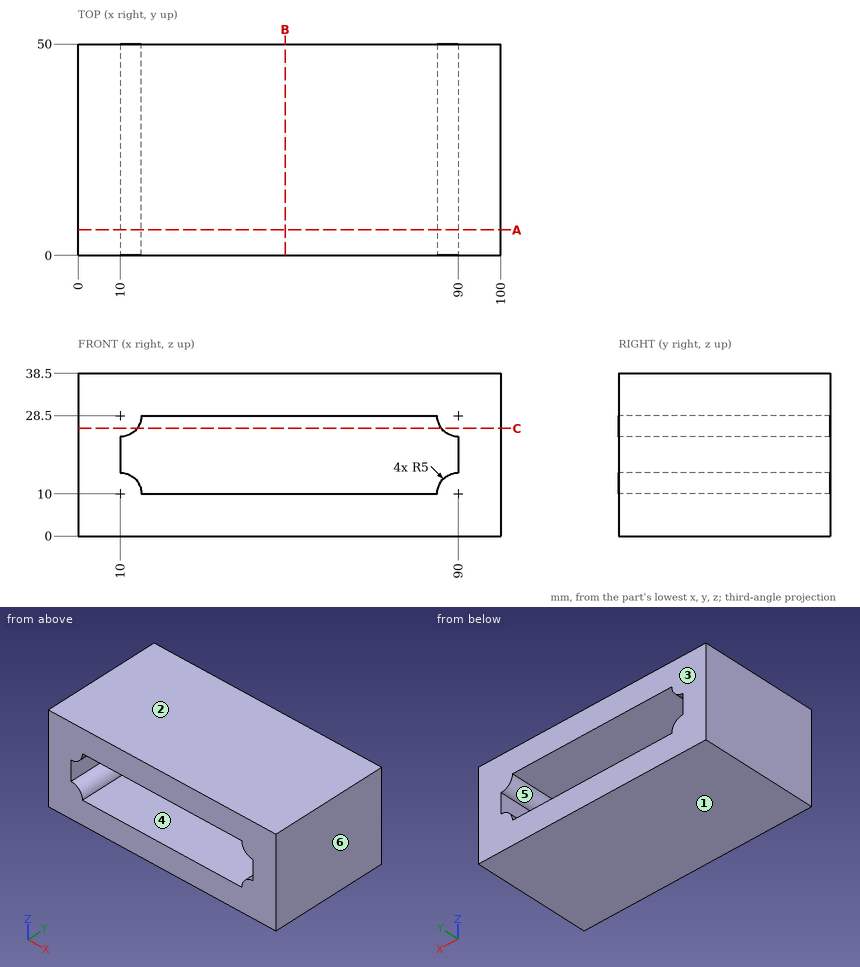
The drawing under review shows one solid part. Ordinate dimensions are in mm from its lowest x, y, z. A direction names the side the tool comes from. Round coordinates to 2 decimals unless told otherwise and drop trailing zeros. Write each loop counter-clockwise with the first axis right and the second up, starting at its lowest first coordinate (ties: lowest second). Pieces come first, ordered by that corner, then holes.
(1) Machinability: for the marked faces 5 and 6, which of the approach directions +Z, -Z, +X, -X, +Y, -Y give a long, thin tool a straight path to every point of the face, cutting with its end or side? Answer none if there is none.
(2) We need section B-B on x = 49. Give the boundary of the cut face in (y, z).
(3) We need section A-A on y = 6. Give the boundary of the cut face in (x, z), and give its area (3 significant figures).
(4) Mouldability with a two-part tool opening along Z and no side actions: class the marked faces 1, 2, 3 and 4 as +Z half, -Z half, draft (parallel to the pull), parting line (faces both ways), or undercut.
(5) Wall thickness on L1, parallel to Z at x = 42.5, y = 10; L2, parallel to X at y = 8, z = 12; L3, parallel to X at y = 17, z = 17: over which ranges is each line inside the solid? List them lowest first.
(6) We need section C-C on z = 25.5. Give the boundary of the cut face in (x, y), and give its area (3 significant figures).
Findings below:
1. face 5: +Y, -Y
1. face 6: +Z, -Z, +X, +Y, -Y
2. outline: (0, 0) - (50, 0) - (50, 10) - (0, 10) - close; (0, 28.5) - (50, 28.5) - (50, 38.5) - (0, 38.5) - close
3. outline: (0, 0) - (100, 0) - (100, 38.5) - (0, 38.5) - close; hole (10, 15) arc R5 cw to (15, 10) - (85, 10) arc R5 cw to (90, 15) - (90, 23.5) arc R5 cw to (85, 28.5) - (15, 28.5) arc R5 cw to (10, 23.5) - close
3. area: 2,450 mm2
4. face 1: -Z half
4. face 2: +Z half
4. face 3: draft
4. face 4: undercut
5. L1: z = 0 to 10, 28.5 to 38.5
5. L2: x = 0 to 14.58, 85.42 to 100
5. L3: x = 0 to 10, 90 to 100
6. outline: (0, 0) - (14, 0) - (14, 50) - (0, 50) - close; (86, 0) - (100, 0) - (100, 50) - (86, 50) - close
6. area: 1,400 mm2
